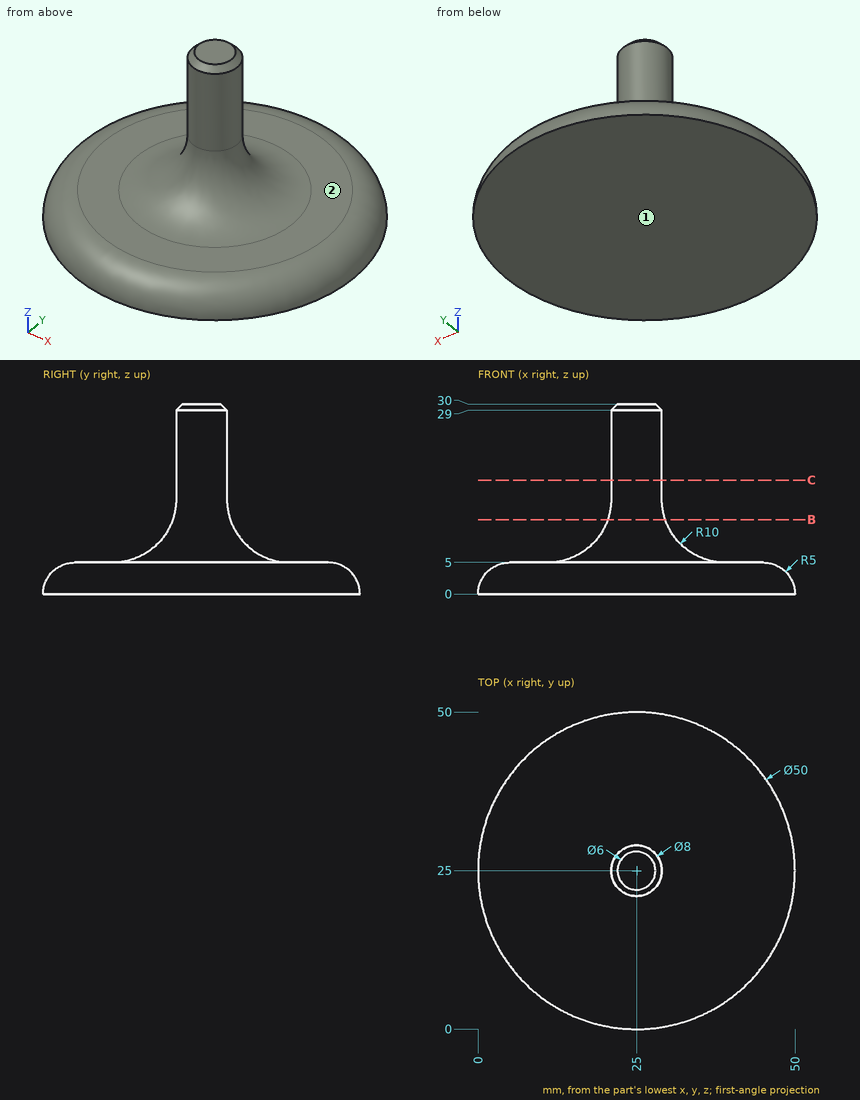
Drawing for the job (mm, zero at the part's lowest x, y, z). A direction names the side the tool comes from. Coordinates: 2 decimals unless noted, no trailing zeros. Write each loop counter-clockwise with the first axis right and the second up, starting at its lowest first coordinate (ties: lowest second). Pieces come first, ordered by that corner, then holes. Notation, with made-up numbers: (11.5, 26.25) -> (67.5, 26.25) arc R27 cw to (67.5, 51.25) -> close; hole circle Ø4 at (-3.75, 67.5). An arc over 180 degrees is marked (long way). One line per item, written item: value. Start each with the question number.
1) Flat gauge pins, fed straight in: pin 1 Ø3 at (x, y) = (13, 26) entering from +Z; pin 2 Ø6 at (x, z) = (25.5, 7.5) entering from -Y. Where does each tip first touch, or does it go through?
2) Probe probe 1 along Z at (x, y) = (9, 20); probe 2 along Y at (x, z) = (10.5, 3.75); probe 3 along Z at (x, y) = (20.5, 21). List the from-to ranges inside material, lowest first.
3) Slice it at C-C on z = 18. Write the cut outline in (x, y).
4) Which spindle directions (+Z, -Z, +X, -X, +Y, -Y) get a long thin tool onto all of the face, cutting with end or side? Do the marked faces 1 and 2. Say none if no direction does.
5) Slice it at B-B on z = 11.75. Write the cut outline in (x, y), then the cut area to 3 significant figures.
Answers follow:
1. pin 1: z = 5.62
1. pin 2: y = 2.83
2. probe 1: 0 to 5
2. probe 2: 6.75 to 43.25
2. probe 3: 0 to 8.97
3. outline: circle Ø8 at (25, 25)
4. face 1: -Z, +X, -X, +Y, -Y
4. face 2: +Z
5. outline: circle Ø9.09 at (25, 25)
5. area: 64.8 mm2
